Autodesk Inventor part; units mm, degrees
ref_plane "YZ Plane" through (0, 0, 0) normal (1, 0, 0) x (0, 1, 0)
ref_plane "XZ Plane" through (0, 0, 0) normal (0, 1, 0) x (-1, 0, 0)
ref_plane "XY Plane" through (0, 0, 0) normal (0, 0, 1) x (1, 0, 0)
sketch "Sketch1" plane through (0, 0, 0) normal (0, 0, 1) x (1, 0, 0)
  line L0 (0, 0) -> (160, 0)
  line L1 (160, 0) -> (160, 160)
  line L2 (160, 160) -> (0, 160)
  line L3 (0, 160) -> (0, 0)
  dimension "d0" = 160
  dimension "d1" = 160
extrude "Extrusion1" add sketch "Sketch1" along normal blind 10
sketch "Sketch2" plane through (0, 0, 10) normal (0, 0, 1) x (1, 0, 0)
  line L0 (0, 160) -> (0, 0)
  line L1 (0, 0) -> (10, 0)
  line L2 (0, 0) -> (160, 0)
  line L3 (10, 0) -> (10, 150)
  line L4 (10, 150) -> (150, 150)
  line L5 (150, 150) -> (150, 10)
  line L6 (150, 10) -> (10, 10)
  line L7 (0, 0) -> (0, 10)
  line L8 (0, 0) -> (0, 2)
  line L9 (160, 160) -> (0, 160)
  line L10 (0, 160) -> (0, 121.5)
  line L11 (0, 160) -> (0, 80)
  line L12 (0, 80) -> (38.5, 80)
  circle A0 centre (38.5, 80) radius 5
  line L13 (160, 0) -> (160, 80)
  line L14 (160, 80) -> (130, 80)
  circle A1 centre (130, 80) radius 8.5
  dimension "d4" = 10
  dimension "d5" = 150
  dimension "d6" = 140
  dimension "d7" = 140
  dimension "d8" = 38.5
  dimension "d9" = 80
  dimension "d10" = 38.5
  dimension "d11" = 10
  dimension "d12" = 80
  dimension "d13" = 30
  dimension "d14" = 17
sketch "Sketch3" plane through (0, 0, 10) normal (0, 0, 1) x (1, 0, 0)
  circle A0 centre (10, 10) radius 5
  circle A1 centre (10, 150) radius 5
  circle A2 centre (150, 150) radius 5
  circle A3 centre (150, 10) radius 5
  point P0 (0, 0)
  dimension "d15" = 10
  dimension "d16" = 10
  dimension "d17" = 10
  dimension "d18" = 10
extrude "Extrusion2" cut sketch "Sketch3" against normal through all
extrude "Extrusion3" cut sketch "Sketch2" against normal through all contours A1 | A0
properties part number "cappingsystem 3rd part"
Geometry: final body of the model. Coordinates: model frame, mm. Coordinates: 2 decimals unless noted, no trailing zeros. Loops run counter-clockwise (first coordinate to the right, second up) from the corner with the lowest first, then second, coordinate; pieces in that order, holes last. Notation, with made-up numbers: (-28.5, 7) - (18.5, 7) arc R17 ccw to (18.5, 37) - close; hole circle Ø9 at (83, 53). An arc over 180 degrees is marked (long way). Put each result on its own line as item: value. Start each with the question number.
Q1. Pull-direction query (X, two-part tool) for faces 1 (the flat face through (81, 160, 5)), 2 (the cylindrical face through (146, 147, 5)), 3 (the flat face through (0, 81, 5)); classes: released by +X, released by -X, zero draft, split by the parting line, or undercut.
Q2. Cut plane C-C, the plane x = 38.5. Return loops of the section in (y, z).
Q3. Cut plane B-B, the plane x = 10. Return loops of the section in (y, z).
Q4. Cut plane A-A, the plane y = 80. Return loops of the section in (x, z), and give its area (3 significant figures).
Q5. Cut plane D-D, the plane z = 8.5. Return loops of the section in (x, y).
Q6. Line query: line 1 (Y direction, x = 10, z = 2.5); line 2 (Y direction, x = 151, z = 3.5); line 3 (Y direction, x = 130, z = 8.25). Output: solid intervals per line, ascending.
Filled sheet:
1. face 1: zero draft
1. face 2: undercut
1. face 3: released by -X
2. outline: (0, 0) - (75, 0) - (75, 10) - (0, 10) - close; (85, 0) - (160, 0) - (160, 10) - (85, 10) - close
3. outline: (0, 0) - (5, 0) - (5, 10) - (0, 10) - close; (15, 0) - (145, 0) - (145, 10) - (15, 10) - close; (155, 0) - (160, 0) - (160, 10) - (155, 10) - close
4. outline: (0, 0) - (33.5, 0) - (33.5, 10) - (0, 10) - close; (43.5, 0) - (121.5, 0) - (121.5, 10) - (43.5, 10) - close; (138.5, 0) - (160, 0) - (160, 10) - (138.5, 10) - close
4. area: 1,330 mm²
5. outline: (0, 0) - (160, 0) - (160, 160) - (0, 160) - close; hole circle Ø10 at (10, 10); hole circle Ø10 at (10, 150); hole circle Ø10 at (38.5, 80); hole circle Ø17 at (130, 80); hole circle Ø10 at (150, 10); hole circle Ø10 at (150, 150)
6. line 1: 0 to 5, 15 to 145, 155 to 160
6. line 2: 0 to 5.1, 14.9 to 145.1, 154.9 to 160
6. line 3: 0 to 71.5, 88.5 to 160
